Could you check a few things on this model? Use its own coordinates, in mm. A direction names the side the tool comes from. Round coordinates to 2 decimals unless told otherwise and drop trailing zeros. Loops run counter-clockwise (first coordinate to the right, second up) from the corner with the lowest first, then second, coordinate; pieces in that order, holes last.
from build123d import *

# Parameters (mm, degrees)
SKETCH1_R           = 1.75
BOSS_EXTRUDE1_DEPTH = 20
CUT_EXTRUDE1_DEPTH  = 20
FILLET1_R           = 3
CUT_EXTRUDE5_DEPTH  = 10


with BuildPart() as part:
    # Sketch1 → Boss-Extrude1 (new body)
    with BuildSketch(Plane(origin=(0, 0, 0), x_dir=(1, 0, 0), z_dir=(0, 1, 0))):
        with BuildLine():
            Line((-86, 29), (-86, -29))
            ThreePointArc((-86, -29), (-85.414213562, -30.414213562), (-84, -31))
            Line((-84, -31), (84, -31))
            ThreePointArc((84, -31), (85.414213562, -30.414213562), (86, -29))
            Line((86, -29), (86, 29))
            ThreePointArc((86, 29), (85.414213562, 30.414213562), (84, 31))
            Line((84, 31), (-84, 31))
            ThreePointArc((-84, 31), (-85.414213562, 30.414213562), (-86, 29))
        make_face()
        with Locations(Location((-81, 26, 0), (0, 0, 270))):  # turned: the seam where the file's is
            Circle(SKETCH1_R, mode=Mode.SUBTRACT)
        with Locations(Location((-81, -26, 0), (0, 0, 270))):  # turned: the seam where the file's is
            Circle(SKETCH1_R, mode=Mode.SUBTRACT)
        with Locations(Location((81, -26, 0), (0, 0, 270))):  # turned: the seam where the file's is
            Circle(SKETCH1_R, mode=Mode.SUBTRACT)
        with Locations(Location((81, 26, 0), (0, 0, 270))):  # turned: the seam where the file's is
            Circle(SKETCH1_R, mode=Mode.SUBTRACT)
        with BuildLine():
            Line((84, -23), (80, -23))
            ThreePointArc((80, -23), (78.585786438, -23.585786438), (78, -25))
            Line((78, -25), (78, -29))
            Line((78, -29), (-78, -29))
            Line((-78, -29), (-78, -25))
            ThreePointArc((-78, -25), (-78.585786438, -23.585786438), (-80, -23))
            Line((-80, -23), (-84, -23))
            Line((-84, -23), (-84, 23))
            Line((-84, 23), (-80, 23))
            ThreePointArc((-80, 23), (-78.585786438, 23.585786438), (-78, 25))
            Line((-78, 25), (-78, 29))
            Line((-78, 29), (78, 29))
            Line((78, 29), (78, 25))
            ThreePointArc((78, 25), (78.585786438, 23.585786438), (80, 23))
            Line((80, 23), (84, 23))
            Line((84, 23), (84, -23))
        make_face(mode=Mode.SUBTRACT)
    extrude(amount=BOSS_EXTRUDE1_DEPTH)

    # Sketch2 → Cut-Extrude1 (cut)
    with BuildSketch(Plane(origin=(0, 0, -31), x_dir=(-1, 0, 0), z_dir=(0, 0, -1))):
        with BuildLine():
            Line((-12, 15), (44, 15))
            ThreePointArc((44, 15), (45.414213562, 14.414213562), (46, 13))
            Line((46, 13), (46, -3))
            Line((46, -3), (-14, -3))
            Line((-14, -3), (-14, 13))
            ThreePointArc((-14, 13), (-13.414213562, 14.414213562), (-12, 15))
        make_face()
    extrude(amount=-CUT_EXTRUDE1_DEPTH, mode=Mode.SUBTRACT)

    # Fillet1
    fillet1_edges = [part.edges().sort_by_distance(p)[0] for p in [
        (84, 10, 23),
        (84, 10, -23),
        (78, 10, -29),
        (-78, 10, -29),
        (-84, 10, -23),
        (-84, 10, 23),
        (-78, 10, 29),
        (78, 10, 29),
    ]]
    fillet(fillet1_edges, radius=FILLET1_R)

    # Sketch3 → Cut-Extrude5 (cut)
    with BuildSketch(Plane(origin=(86, 0, 0), x_dir=(0, 0, -1), z_dir=(1, 0, 0))):
        with BuildLine():
            Line((-13, 0), (-13, 6))
            ThreePointArc((-13, 6), (-13.585786438, 7.414213562), (-15, 8))
            Line((-15, 8), (-19, 8))
            ThreePointArc((-19, 8), (-20.414213562, 7.414213562), (-21, 6))
            Line((-21, 6), (-21, 0))
            Line((-21, 0), (-13, 0))
        make_face()
    extrude(amount=-CUT_EXTRUDE5_DEPTH, mode=Mode.SUBTRACT)


solid = part.part
Item 1: If I drill on line 1 along X through (y, z) = (11.75, -26); line 2 along Z through (x, y) = (81, 11.5); line 3 along X through (y, z) = (2, 10), over which ranges is the centre line in solid material (lowest first)?
Results list:
line 1: x = -86 to -82.75, -79.25 to -78, 78 to 79.25, 82.75 to 86
line 2: z = -31 to -27.75, -24.25 to -23, 23 to 24.25, 27.75 to 31
line 3: x = -86 to -84, 84 to 86
Item 2: If we section it at A-A, the plane x = -41: Please give me the cut outline in (y, z).
Results list:
outline: (0, 29) - (20, 29) - (20, 31) - (0, 31) - close; (15, -31) - (20, -31) - (20, -29) - (15, -29) - close
Item 3: For faces 1 (the flat face through (84, 10, 0)), 2 (the flat face through (1, 17, -31)), which set-ups out of +Z, -Z, +X, -X, +Y, -Y let a thin tool reach every point of the face, with its end or its side?
Results list:
face 1: +Y, -Y
face 2: -Z, +X, -X, +Y, -Y
Item 4: If we section it at B-B, the plane z = 10.5: Please give me the cut outline in (x, y).
Results list:
outline: (-86, 0) - (-84, 0) - (-84, 20) - (-86, 20) - close; (84, 0) - (86, 0) - (86, 20) - (84, 20) - close
Item 5: We'd pull the mould along Z, two halves only. Please class faces 3 (the flat face through (-1, 10, 31)), 4 (the flat face through (-86, 10, 0)), 5 (the cylindrical face through (77.1, 10.14, -28.14)): released by +Z, released by -Z, zero draft, split by the parting line, or undercut.
Results list:
face 3: released by +Z
face 4: zero draft
face 5: undercut
Item 6: If we section it at C-C, the plane y = 3.5: Count the separate pieces of the cut face and the enclosed holes in it, then the cut area to 3 significant figures.
Results list:
separate pieces: 2
enclosed holes: 4
area: 898 mm2
Item 7: Will these pins go through, and if not, where does the flat tip stop? pin 1 (8 mm diameter, centred on x = 15.5, z = -23, fed in from +Y); pin 2 (0.6 mm diameter, centred on y = 7.5, z = -30.5, fed in from +X); pin 3 (1.6 mm diameter, centred on x = -27, z = -30, fed in from -Y); pin 4 (5.5 mm diameter, centred on x = -81, z = -26, fed in from -Y).
Results list:
pin 1: passes through
pin 2: stops at x = 85.6
pin 3: stops at y = 15
pin 4: stops at y = 0
